Source: CAD feature listing. Evaluate the final solid. Frame: model axes, mm. A direction names the side the tool comes from. Give positions to 0.01 mm unless a question says otherwise; leave off trailing zeros. Loops run counter-clockwise (first coordinate to the right, second up) from the corner with the lowest first, then second, coordinate; pieces in that order, holes last. Notation, with made-up numbers: (85, 29) - (108, 29) arc R25 cw to (108, 68) - close; hole circle Ø1 at (59, -38.5). An arc over 180 degrees is marked (long way). Put each result on its own line as item: value.
Autodesk Inventor part; units mm, degrees
ref_plane "YZ Plane" through (0, 0, 0) normal (1, 0, 0) x (0, 1, 0)
ref_plane "XZ Plane" through (0, 0, 0) normal (0, 1, 0) x (-1, 0, 0)
ref_plane "XY Plane" through (0, 0, 0) normal (0, 0, 1) x (1, 0, 0)
sketch "Sketch1" plane through (0, 0, 0) normal (0, 1, 0) x (-1, 0, 0)
  line L0 (-125, 50) -> (125, 50)
  line L1 (125, 50) -> (125, -50)
  line L2 (125, -50) -> (-125, -50)
  line L3 (-125, -50) -> (-125, 50)
  line L4 (-125, 50) -> (125, -50) construction
  line L5 (125, 50) -> (-125, -50) construction
  line L6 (0, 50) -> (0, -50) construction
  line L7 (125, 25) -> (130, 25)
  line L8 (130, 25) -> (130, -25)
  line L9 (130, -25) -> (125, -25)
  line L10 (125, -25) -> (125, 25)
  line L11 (-125, 25) -> (-130, 25)
  line L12 (-130, 25) -> (-130, -25)
  line L13 (-130, -25) -> (-125, -25)
  point P0 (0, 0)
  dimension "d0" = 100
  dimension "d1" = 250
  dimension "d2" = 50
  dimension "d3" = 5
  dimension "d4" = 25
extrude "Extrusion1" add sketch "Sketch1" along normal blind 5
equation "\"BendRadius\" = Thickness"
equation "\"BendReliefWidth\" = Thickness"
equation "\"BendReliefDepth\" = 0.5 * Thickness"
equation "\"CornerReliefSize\" = 4 * Thickness"
equation "\"MinimumRemnant\" = 2 * Thickness"
equation "\"TransitionRadius\" = BendRadius"
equation "\"JacobiRadiusSize\" = BendRadius"
equation "\"GapSize\" = Thickness"
properties part number "Tapa2" material "Wood (Cherry)"
1) Material intervals for line 1 along X through (y, z) = (4.2, 43), sorted ascending. Write a range as [from, to].
Check result:
line 1: [-125, 125]
2) Pin query (flat end, axial travel): P1, Ø3, axis at y = 2.5, z = -38, coming from the +X side; P2, Ø1.5, axis at x = 128, y = 3, coming from the +Z side. Return the tip coordinate at first contact, or that it passes through.
Check result:
P1: x = 125
P2: z = 25
3) Access query for faces 1 (the flat face through (125, 2, 37)), 2 (the flat face through (-127, 2, 25)), 3 (the flat face through (-128, 2, -25)), 4 (the flat face through (2, 0, 1)), 5 (the flat face through (125, 2, -38)). Directions: +Z, -Z, +X, -X, +Y, -Y. A direction counts if a zero-diameter tool reaches every point of the face in a straight line with its end or side. Return the directions, or none.
Check result:
face 1: +Z, +X, +Y, -Y
face 2: +Z, -X, +Y, -Y
face 3: -Z, -X, +Y, -Y
face 4: +Z, -Z, +X, -X, -Y
face 5: -Z, +X, +Y, -Y
4) Section query B-B, the plane z = 35. Output: boundary loops of the cut face in (x, y).
Check result:
outline: (-125, 0) - (125, 0) - (125, 5) - (-125, 5) - close
5) Section query A-A, the plane y = 2.65. Output: boundary loops of the cut face in (x, z).
Check result:
outline: (-130, -25) - (-125, -25) - (-125, -50) - (125, -50) - (125, -25) - (130, -25) - (130, 25) - (125, 25) - (125, 50) - (-125, 50) - (-125, 25) - (-130, 25) - close
